Read the model definition and answer for the solid it produces. Units are mm, in the model's axes. A direction names the side the tool comes from. Coordinates: 2 decimals unless noted, no trailing zeros. Loops run counter-clockwise (first coordinate to the right, second up) from the corner with the lowest first, then second, coordinate; pieces in that order, holes last.
Q1. The mould has two halves that part along Y. Classify faces 5 (the face through (38, -38, -508)), 6 (the face through (188, 0, 125)), 7 (the face through (283, -378.46, 127)): pulls with the +Y half, pulls with the -Y half, needs draft (parallel to the pull), parting line crosses it, or undercut.
Q2. Section C-C (x = 246) is taken. Give the vertices of the cut face in (y, z), then the cut area to 3 significant figures.
Q3. Section B-B (z = 133) is taken. Give the vertices of the cut face in (x, y), then the cut area to 3 significant figures.
Q4. Section A-A (z = -27.5) is taken. Give the vertices of the cut face in (x, y), then the cut area to 3 significant figures.
Q5. Which of the six approach directions +Z, -Z, +X, -X, +Y, -Y give full straight-line access (tool end or side, diameter ignored) to faces 1 (the face through (330.2, -38, -250)), 2 (the face through (378.46, -193, 127)), 3 (the face through (355.6, -343, -250)), 4 (the face through (25.4, -343, -250))?
Q6. Flat-ended cylindrical pins translate along their axes: P1, Ø10, axis at y = -103.5, z = -9.5, coming from the +X side; P2, Ø6, axis at y = -331, z = -79, coming from the -X side; P3, Ø5, axis at x = 269, y = -295.5, coming from the -Z side; P4, Ø20.5, axis at y = -344, z = -366, coming from the +X side. Find the tip coordinate at first contact, or state that the pin passes through.
Q7. Section D-D (y = -294) is taken. Give the vertices of the cut face in (x, z), then the cut area to 3 significant figures.
Q8. Straight lines are drawn through the part: line 1 (X direction, y = -25.5, z = -358); line 2 (Y direction, x = 92, z = 95); line 3 (Z direction, x = 242.5, y = -184). For each, find the intervals that lie inside material, in ascending order.
from build123d import *

# Parameters (mm, degrees)
F0_W     = 381
F0_H     = 381
F1_DEPTH = 254
F2_T     = -2.54
F3_W     = 25.4
F3_H     = 25.4
F4_DEPTH = 508
F5_W     = 6.35
F5_H     = 375.92
F6_DEPTH = 254


with BuildPart() as f1:
    # F0 (on Top) → F1 (new body)
    with BuildSketch(Plane.XY):
        with Locations((190.5, -190.5)):
            Rectangle(F0_W, F0_H)
    extrude(amount=F1_DEPTH)

    # F2
    f2_openings = [f1.faces().sort_by_distance(p)[0] for p in [
        (190.5, -190.5, 254),
    ]]
    offset(amount=F2_T, openings=f2_openings)

    # F3 (on face) → F4 (join)
    with BuildSketch(Plane(origin=(0, 0, 0), x_dir=(1, 0, 0), z_dir=(0, 0, -1))):
        with Locations((38.1, 342.9)):
            Rectangle(F3_W, F3_H)
        with Locations((342.9, 342.9)):
            Rectangle(F3_W, F3_H)
        with Locations((38.1, 38.1)):
            Rectangle(F3_W, F3_H)
        with Locations((342.9, 38.1)):
            Rectangle(F3_W, F3_H)
    extrude(amount=F4_DEPTH)

    # F5 (on face) → F6 (join)
    with BuildSketch(Plane.XY.offset(2.54)):
        with Locations((187.325, -190.5)):
            Rectangle(F5_W, F5_H)
    extrude(amount=F6_DEPTH)


solid = f1.part
Numbers:
1. face 5: needs draft
1. face 6: pulls with the +Y half
1. face 7: undercut
2. outline: (-381, 0) - (0, 0) - (0, 254) - (-2.54, 254) - (-2.54, 2.54) - (-378.46, 2.54) - (-378.46, 254) - (-381, 254) - close
2. area: 2,250 mm2
3. outline: (0, -381) - (381, -381) - (381, 0) - (0, 0) - close; hole (2.54, -378.46) - (184.15, -378.46) - (184.15, -2.54) - (2.54, -2.54) - close; hole (190.5, -378.46) - (378.46, -378.46) - (378.46, -2.54) - (190.5, -2.54) - close
3. area: 6,230 mm2
4. outline: (25.4, -355.6) - (50.8, -355.6) - (50.8, -330.2) - (25.4, -330.2) - close; (25.4, -50.8) - (50.8, -50.8) - (50.8, -25.4) - (25.4, -25.4) - close; (330.2, -355.6) - (355.6, -355.6) - (355.6, -330.2) - (330.2, -330.2) - close; (330.2, -50.8) - (355.6, -50.8) - (355.6, -25.4) - (330.2, -25.4) - close
4. area: 2,580 mm2
5. face 1: -Z, +Y, -Y
5. face 2: +Z
5. face 3: -Z, +X, +Y, -Y
5. face 4: -Z, -X, +Y, -Y
6. P1: passes through
6. P2: stops at x = 25.4
6. P3: stops at z = 0
6. P4: stops at x = 355.6
7. outline: (0, 0) - (381, 0) - (381, 254) - (378.46, 254) - (378.46, 2.54) - (190.5, 2.54) - (190.5, 256.54) - (184.15, 256.54) - (184.15, 2.54) - (2.54, 2.54) - (2.54, 254) - (0, 254) - close
7. area: 3,860 mm2
8. line 1: x = 25.4 to 50.8, 330.2 to 355.6
8. line 2: y = -381 to -378.46, -2.54 to 0
8. line 3: z = 0 to 2.54
